The listing builds one solid part. Answer for the finished solid, in the listing's coordinates (mm). Coordinates: 2 decimals unless noted, no trailing zeros. Order: outer loops, then holes, each group sorted by start corner. A loop starts at its lowest first (then second) coordinate and runs counter-clockwise, first axis right, second up. Notation, with made-up numbers: (66.25, 45) -> (95.25, 45) arc R33 cw to (95.25, 76) -> close; hole circle Ø6 at (72.25, 81.5). An arc over 180 degrees is marked (long way). Return JSON: item names as keys, results as strings.
from build123d import *

# Parameters (mm, degrees)
SKETCH_1_R      = 2.1
EXTRUDE_1_DEPTH = 100
VERRUNDUNG1_R   = 1


with BuildPart() as part:
    # 草图1 → 凸台-拉伸1 (new body)
    with BuildSketch(Plane.XY):
        Polygon((5.71, 20), (-5.71, 20), (-6.9, 18.81), (-6.9, 18.2), (-4.5, 18.2), (-4.5, 16.489949494), (-7.089949494, 13.9), (-12.910050506, 13.9), (-15.5, 16.489949494), (-15.5, 18.2), (-13.1, 18.2), (-13.1, 18.81), (-14.29, 20), (-20, 20), (-20, 14.29), (-18.81, 13.1), (-18.2, 13.1), (-18.2, 15.5), (-16.489949494, 15.5), (-13.9, 12.910050506), (-13.9, 7.089949494), (-16.489949494, 4.5), (-18.2, 4.5), (-18.2, 6.9), (-18.81, 6.9), (-20, 5.71), (-20, -5.71), (-18.81, -6.9), (-18.2, -6.9), (-18.2, -4.5), (-16.489949494, -4.5), (-13.9, -7.089949494), (-13.9, -12.910050506), (-16.489949494, -15.5), (-18.2, -15.5), (-18.2, -13.1), (-18.81, -13.1), (-20, -14.29), (-20, -20), (-14.29, -20), (-13.1, -18.81), (-13.1, -18.2), (-15.5, -18.2), (-15.5, -16.489949494), (-12.910050506, -13.9), (-7.089949494, -13.9), (-4.5, -16.489949494), (-4.5, -18.2), (-6.9, -18.2), (-6.9, -18.81), (-5.71, -20), (5.71, -20), (6.9, -18.81), (6.9, -18.2), (4.5, -18.2), (4.5, -16.489949494), (7.089949494, -13.9), (12.910050506, -13.9), (15.5, -16.489949494), (15.5, -18.2), (13.1, -18.2), (13.1, -18.81), (14.29, -20), (20, -20), (20, -14.29), (18.81, -13.1), (18.2, -13.1), (18.2, -15.5), (16.489949494, -15.5), (13.9, -12.910050506), (13.9, -7.089949494), (16.489949494, -4.5), (18.2, -4.5), (18.2, -6.9), (18.81, -6.9), (20, -5.71), (20, 5.71), (18.81, 6.9), (18.2, 6.9), (18.2, 4.5), (16.489949494, 4.5), (13.9, 7.089949494), (13.9, 12.910050506), (16.489949494, 15.5), (18.2, 15.5), (18.2, 13.1), (18.81, 13.1), (20, 14.29), (20, 20), (14.29, 20), (13.1, 18.81), (13.1, 18.2), (15.5, 18.2), (15.5, 16.489949494), (12.910050506, 13.9), (7.089949494, 13.9), (4.5, 16.489949494), (4.5, 18.2), (6.9, 18.2), (6.9, 18.81), align=None)
        with Locations((-10, 10)):
            Circle(SKETCH_1_R, mode=Mode.SUBTRACT)
        with Locations(Location((-10, -10, 0), (0, 0, 180))):
            Circle(SKETCH_1_R, mode=Mode.SUBTRACT)
        with Locations((10, -10)):
            Circle(SKETCH_1_R, mode=Mode.SUBTRACT)
        with Locations(Location((10, 10, 0), (0, 0, 180))):
            Circle(SKETCH_1_R, mode=Mode.SUBTRACT)
        Polygon((-6.1, 6.1), (-6.1, 12.910050506), (-3, 16.010050506), (-3, 18.2), (3, 18.2), (3, 16.010050506), (6.1, 12.910050506), (6.1, 6.1), (12.910050506, 6.1), (16.010050506, 3), (18.2, 3), (18.2, -3), (16.010050506, -3), (12.910050506, -6.1), (6.1, -6.1), (6.1, -12.910050506), (3, -16.010050506), (3, -18.2), (-3, -18.2), (-3, -16.010050506), (-6.1, -12.910050506), (-6.1, -6.1), (-12.910050506, -6.1), (-16.010050506, -3), (-18.2, -3), (-18.2, 3), (-16.010050506, 3), (-12.910050506, 6.1), align=None, mode=Mode.SUBTRACT)
    extrude(amount=EXTRUDE_1_DEPTH)

    # Verrundung1
    verrundung1_edges = [part.edges().sort_by_distance(p)[0] for p in [
        (20, 20, 50),
        (20, -20, 50),
        (-20, -20, 50),
        (-20, 20, 50),
    ]]
    fillet(verrundung1_edges, radius=VERRUNDUNG1_R)


solid = part.part
1. The part is cut by section B-B on x = 10. Give the vertices of the cut face in (y, z).
Answer block:
{"outline": "(-13.9, 0) -> (-12.1, 0) -> (-12.1, 100) -> (-13.9, 100) -> close; (-7.9, 0) -> (-6.1, 0) -> (-6.1, 100) -> (-7.9, 100) -> close; (6.1, 0) -> (7.9, 0) -> (7.9, 100) -> (6.1, 100) -> close; (12.1, 0) -> (13.9, 0) -> (13.9, 100) -> (12.1, 100) -> close"}
2. Each of these flat-tipped pins is pushed along its axis until it touches: pin 1 Ø7.5 at (y, z) = (10, 39.5) entering from +X; pin 2 Ø1.7 at (y, z) = (10.5, 42.5) entering from +X; pin 3 Ø1.5 at (x, z) = (-11, 45.5) entering from +Y; pin 4 Ø8 at (x, y) = (0, -6) entering from +Z. Where does it stop, or does it pass through?
Answer block:
{"pin 1": "stops at x = 19.46", "pin 2": "stops at x = 13.9", "pin 3": "stops at y = 13.9", "pin 4": "passes through"}
3. The part is cut by section A-A on y = -0.5. Give the vertices of the cut face in (x, z), and give its area (3 significant figures).
Answer block:
{"outline": "(-20, 0) -> (-18.2, 0) -> (-18.2, 100) -> (-20, 100) -> close; (18.2, 0) -> (20, 0) -> (20, 100) -> (18.2, 100) -> close", "area": "360 mm2"}
4. Consider line 1 (Y direction, x = 10, z = 26); line 2 (Y direction, x = -16.5, z = 29.5); line 3 (X direction, y = -2, z = 54). Determine where each line is inside the solid, lowest interval first. Write a range as from..to.
Answer block:
{"line 1": "y = -13.9..-12.1, -7.9..-6.1, 6.1..7.9, 12.1..13.9", "line 2": "y = -20..-15.5, -4.5..-3, 3..4.5, 15.5..20", "line 3": "x = -20..-18.2, 18.2..20"}
5. Determine the mould class of faces 1 (the face through (-20, 17, 49)), 2 (the face through (-12.1, 10.09, 49.3)), 3 (the face through (-17, -20, 49)) for opening direction Y: pulls with the +Y half, pulls with the -Y half, needs draft (parallel to the pull), parting line crosses it, or undercut.
Answer block:
{"face 1": "needs draft", "face 2": "undercut", "face 3": "pulls with the -Y half"}
